```python
from build123d import *

# Parameters (mm, degrees)
FILLET1_R           = 0.127
SKETCH2_R           = 6.35
BOSS_EXTRUDE1_DEPTH = 3.81
SKETCH3_R           = 3.175
CUT_EXTRUDE1_DEPTH  = 24.992209055


with BuildPart() as part:
    # Sketch1 → Revolve1 (revolve)
    with BuildSketch(Plane.XY, mode=Mode.PRIVATE) as revolve1_sk:
        with BuildLine():
            Line((-1.905, 0), (-1.905, 16.51))
            Line((-1.905, 16.51), (-1.070224719, 14.797640449))
            ThreePointArc((-1.070224719, 14.797640449), (0, 14.12875), (1.070224719, 14.797640449))
            Line((1.070224719, 14.797640449), (1.905, 16.51))
            Line((1.905, 16.51), (1.905, 0))
            Line((1.905, 0), (-1.905, 0))
        make_face()
    revolve(revolve1_sk.sketch.rotate(Axis((-602.921612104, 0, 0), (1, 0, 0)), 90), axis=Axis((-602.921612104, 0, 0), (1, 0, 0)))

    # Fillet1
    fillet1_edges = [part.edges().sort_by_distance(p)[0] for p in [
        (1.905, 0, -16.51),
        (-1.905, 0, -16.51),
    ]]
    fillet(fillet1_edges, radius=FILLET1_R)

    # Sketch2 → Boss-Extrude1 (add)
    with BuildSketch(Plane(origin=(1.905, 0, 0), x_dir=(0, 0, -1), z_dir=(1, 0, 0))):
        with Locations(Location((0, 0, 0), (0, 0, 180))):
            Circle(SKETCH2_R)
    extrude(amount=BOSS_EXTRUDE1_DEPTH)

    # Sketch3 → Cut-Extrude1 (cut, through all)
    with BuildSketch(Plane(origin=(5.715, 0, 0), x_dir=(0, 0, -1), z_dir=(1, 0, 0))):
        Circle(SKETCH3_R)
    extrude(amount=-CUT_EXTRUDE1_DEPTH, mode=Mode.SUBTRACT)


solid = part.part
```
For this review, take the finished solid that the model builds, in its own axes (mm). A direction names the side the tool comes from. Round coordinates to 2 decimals unless told otherwise and drop trailing zeros. Write each loop counter-clockwise with the first axis right and the second up, starting at its lowest first coordinate (ties: lowest second). Pieces come first, ordered by that corner, then holes. Notation, with made-up numbers: (16.5, 22.25) -> (27.5, 22.25) arc R15 ccw to (27.5, 44.25) -> close; hole circle Ø10 at (39, -13.75). An arc over 180 degrees is marked (long way). Use one line per item in the form item = value.
Q1. Machinability: for faces 4 (the cylindrical face through (1.96, -3.1, 0.69)), 5 (the flat face through (1.905, 0, 7)), which of the approach directions +Z, -Z, +X, -X, +Y, -Y give a long, thin tool a straight path to every point of the face, cutting with its end or side? Answer none if there is none.
Resolved:
face_4 = +X, -X
face_5 = +X
Q2. To check wall thickness, follow probe 1 along Y at (x, z) = (2.5, 0) (3 decimals); probe 2 along X at (y, z) = (-11, -8.5) (3 decimals); probe 3 along Y at (x, z) = (1.5, 0) (3 decimals). State the ranges of each line that lie inside material, in increasing order. Write a range as from..to.
Resolved:
probe_1 = -6.35..-3.175, 3.175..6.35
probe_2 = -1.905..1.905
probe_3 = -15.679..-3.175, 3.175..15.679
Q3. The part is to be moulded in two halves that separate along X. For faces 1 (the flat face through (-1.905, -0.22, -3.32)), 2 (the cylindrical face through (3.783, 5.634, 2.93)), 3 (the flat face through (5.715, -3, -2)), say which applies: released by +X, released by -X, zero draft, split by the parting line, or undercut.
Resolved:
face_1 = released by -X
face_2 = zero draft
face_3 = released by +X
Q4. Consider section D-D (x = -0.25). State the section outline as (y, z) points (3 decimals), then the cut area to 3 significant figures.
Resolved:
outline = circle Ø28.311 at (0, 0); hole circle Ø6.35 at (0, 0)
area = 598 mm²
Q5. Clearance check with flat-ended pins moving along their axes: pin 1 Ø5 at (y, z) = (9, -11) entering from +X (3 decimals); pin 2 Ø3 at (x, z) = (2, 3.5) entering from -Y. State where each tip first meets the part, or that it passes through.
Resolved:
pin_1 = 1.905
pin_2 = -15.96
Q6. Consider section C-C (x = 4.25). State the section outline as (y, z) points (3 decimals).
Resolved:
outline = circle Ø12.7 at (0, 0); hole circle Ø6.35 at (0, 0)
Q7. Consider section A-A (y = 0). State the section outline as (x, z) points (3 decimals), then the cut area to 3 significant figures.
Resolved:
outline = (-1.905, -15.96) arc R0.127 ccw to (-1.664, -16.015) -> (-1.07, -14.798) arc R1.191 cw to (1.07, -14.798) -> (1.664, -16.015) arc R0.127 ccw to (1.905, -15.96) -> (1.905, -6.35) -> (5.715, -6.35) -> (5.715, -3.175) -> (-1.905, -3.175) -> close; (-1.905, 3.175) -> (5.715, 3.175) -> (5.715, 6.35) -> (1.905, 6.35) -> (1.905, 15.96) arc R0.127 ccw to (1.664, 16.015) -> (1.07, 14.798) arc R1.191 cw to (-1.07, 14.798) -> (-1.664, 16.015) arc R0.127 ccw to (-1.905, 15.96) -> close
area = 113 mm²
